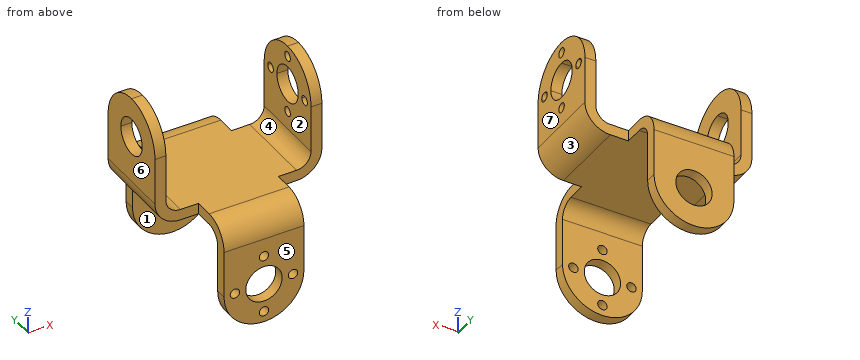
from build123d import *

# Parameters (mm, degrees)
BOSS_EXTRUDE1_DEPTH  = 3
BOSS_EXTRUDE2_DEPTH  = 22
BOSS_EXTRUDE10_DEPTH = 22
BOSS_EXTRUDE3_START  = 3
SKETCH3_R            = 1.3
SKETCH3_R_2          = 5
BOSS_EXTRUDE3_DEPTH  = 3
SKETCH5_W            = 32
SKETCH5_H            = 22
BOSS_EXTRUDE4_DEPTH  = 3
BOSS_EXTRUDE5_DEPTH  = 22
SKETCH8_R            = 1.3
BOSS_EXTRUDE8_DEPTH  = 3
BOSS_EXTRUDE9_START  = -3
BOSS_EXTRUDE9_DEPTH  = 3


with BuildPart() as part:
    # Sketch1 → Boss-Extrude1 (new body)
    with BuildSketch(Plane(origin=(0, 0, 0), x_dir=(1, 0, 0), z_dir=(0, 1, 0))):
        with BuildLine():
            ThreePointArc((-5, 0), (0, 5), (5, 0))
            Line((5, 0), (11, 0))
            ThreePointArc((11, 0), (0, 11), (-11, 0))
            Line((-11, 0), (-5, 0))
        make_face()
        with BuildLine():
            Line((11, 0), (5, 0))
            ThreePointArc((5, 0), (0, -5), (-5, 0))
            Line((-5, 0), (-11, 0))
            ThreePointArc((-11, 0), (0, -11), (11, 0))
        make_face()
        with BuildLine():
            Line((11, -13), (11, 0))
            ThreePointArc((11, 0), (0, -11), (-11, 0))
            Line((-11, 0), (-11, -13))
            Line((-11, -13), (11, -13))
        make_face()
    extrude(amount=BOSS_EXTRUDE1_DEPTH)

    # Sketch2 → Boss-Extrude2 (add)
    with BuildSketch(Plane(origin=(11, 0, 0), x_dir=(0, 0, -1), z_dir=(1, 0, 0))):
        with BuildLine():
            Line((-13, 0), (-13, 3))
            ThreePointArc((-13, 3), (-17.949747468, 0.949747468), (-20, -4))
            Line((-20, -4), (-20, -36))
            Line((-20, -36), (-17, -36))
            Line((-17, -36), (-17, -4))
            ThreePointArc((-17, -4), (-15.828427125, -1.171572875), (-13, 0))
        make_face()
    extrude(amount=-BOSS_EXTRUDE2_DEPTH)

    # Sketch2<4> → Boss-Extrude10 (add)
    with BuildSketch(Plane(origin=(11, 0, 0), x_dir=(0, 0, -1), z_dir=(1, 0, 0))):
        with BuildLine():
            Line((-20, -36), (-17, -36))
            ThreePointArc((-17, -36), (-15.828427125, -38.828427125), (-13, -40))
            Line((-13, -40), (-13, -43))
            ThreePointArc((-13, -43), (-17.949747468, -40.949747468), (-20, -36))
        make_face()
    extrude(amount=-BOSS_EXTRUDE10_DEPTH)

    # Sketch3 → Boss-Extrude3 (add)
    with BuildSketch(Plane(origin=(0, -40, 0), x_dir=(-1, 0, 0), z_dir=(0, -1, 0)).offset(BOSS_EXTRUDE3_START)):
        with BuildLine():
            ThreePointArc((11, 0), (0, 11), (-11, 0))
            Line((-11, 0), (-11, -13))
            Line((-11, -13), (11, -13))
            Line((11, -13), (11, 0))
        make_face()
        with Locations(Location((8, 0, 0), (0, 0, 90))):
            Circle(SKETCH3_R, mode=Mode.SUBTRACT)
        with Locations(Location((0, 0, 0), (0, 0, 270))):
            Circle(SKETCH3_R_2, mode=Mode.SUBTRACT)
        with Locations(Location((-8, 0, 0), (0, 0, 90))):
            Circle(SKETCH3_R, mode=Mode.SUBTRACT)
        with Locations(Location((0, 8, 0), (0, 0, 90))):
            Circle(SKETCH3_R, mode=Mode.SUBTRACT)
        with Locations(Location((0, -8, 0), (0, 0, 90))):
            Circle(SKETCH3_R, mode=Mode.SUBTRACT)
    extrude(amount=-BOSS_EXTRUDE3_DEPTH)

    # Sketch5 → Boss-Extrude4 (add)
    with BuildSketch(Plane.XY.offset(20)):
        with Locations((0, -20)):
            Rectangle(SKETCH5_W, SKETCH5_H)
    extrude(amount=-BOSS_EXTRUDE4_DEPTH)

    # Sketch6 → Boss-Extrude5 (add)
    with BuildSketch(Plane(origin=(0, -9, 0), x_dir=(1, 0, 0), z_dir=(0, 1, 0))):
        with BuildLine():
            Line((-23, -24), (-20, -24))
            ThreePointArc((-20, -24), (-18.828427125, -21.171572875), (-16, -20))
            Line((-16, -20), (-16, -17))
            ThreePointArc((-16, -17), (-20.949747468, -19.050252532), (-23, -24))
        make_face()
        with BuildLine():
            Line((20, -24), (23, -24))
            ThreePointArc((23, -24), (20.949747468, -19.050252532), (16, -17))
            Line((16, -17), (16, -20))
            ThreePointArc((16, -20), (18.828427125, -21.171572875), (20, -24))
        make_face()
    extrude(amount=-BOSS_EXTRUDE5_DEPTH)

    # Sketch8 → Boss-Extrude8 (add)
    # profile 1 of 3: a face of its own
    with BuildSketch(Plane.ZY.offset(-23)):
        with BuildLine():
            Line((37, -9), (24, -9))
            Line((24, -9), (24, -31))
            Line((24, -31), (37, -31))
            ThreePointArc((37, -31), (26, -20), (37, -9))
        make_face()
    # profile 2 of 3: a face of its own
    with BuildSketch(Plane.ZY.offset(-23)):
        with BuildLine():
            Line((37, -10.7), (37, -9))
            ThreePointArc((37, -9), (26, -20), (37, -31))
            Line((37, -31), (37, -29.3))
            ThreePointArc((37, -29.3), (35.7, -28), (37, -26.7))
            Line((37, -26.7), (37, -25))
            ThreePointArc((37, -25), (32, -20), (37, -15))
            Line((37, -15), (37, -13.3))
            ThreePointArc((37, -13.3), (35.7, -12), (37, -10.7))
        make_face()
        with Locations((29, -20)):
            Circle(SKETCH8_R, mode=Mode.SUBTRACT)
    # profile 3 of 3: a face of its own
    with BuildSketch(Plane.ZY.offset(-23)):
        with BuildLine():
            ThreePointArc((48, -20), (44.778174593, -12.221825407), (37, -9))
            Line((37, -9), (37, -10.7))
            ThreePointArc((37, -10.7), (37.919238816, -11.080761184), (38.3, -12))
            ThreePointArc((38.3, -12), (37.919238816, -12.919238816), (37, -13.3))
            Line((37, -13.3), (37, -15))
            ThreePointArc((37, -15), (40.535533906, -16.464466094), (42, -20))
            ThreePointArc((42, -20), (40.535533906, -23.535533906), (37, -25))
            Line((37, -25), (37, -26.7))
            ThreePointArc((37, -26.7), (37.919238816, -27.080761184), (38.3, -28))
            ThreePointArc((38.3, -28), (37.919238816, -28.919238816), (37, -29.3))
            Line((37, -29.3), (37, -31))
            ThreePointArc((37, -31), (44.778174593, -27.778174593), (48, -20))
        make_face()
        with Locations((45, -20)):
            Circle(SKETCH8_R, mode=Mode.SUBTRACT)
    extrude(amount=BOSS_EXTRUDE8_DEPTH)

    # Sketch9 → Boss-Extrude9 (add)
    with BuildSketch(Plane.ZY.offset(23).offset(BOSS_EXTRUDE9_START)):
        with BuildLine():
            Line((24, -9), (24, -31))
            Line((24, -31), (37, -31))
            ThreePointArc((37, -31), (26, -20), (37, -9))
            Line((37, -9), (24, -9))
        make_face()
        with BuildLine():
            ThreePointArc((37, -9), (26, -20), (37, -31))
            Line((37, -31), (37, -25))
            ThreePointArc((37, -25), (32, -20), (37, -15))
            Line((37, -15), (37, -9))
        make_face()
        with BuildLine():
            Line((37, -25), (37, -31))
            ThreePointArc((37, -31), (44.778174593, -27.778174593), (48, -20))
            ThreePointArc((48, -20), (44.778174593, -12.221825407), (37, -9))
            Line((37, -9), (37, -15))
            ThreePointArc((37, -15), (40.535533906, -16.464466094), (42, -20))
            ThreePointArc((42, -20), (40.535533906, -23.535533906), (37, -25))
        make_face()
    extrude(amount=BOSS_EXTRUDE9_DEPTH)


solid = part.part
Build history of the part. All positions in model axes, mm. Face numbers are marked on the shaded views. A direction names the side the tool comes from. Coordinates: 2 decimals unless noted, no trailing zeros. Order: outer loops, then holes, each group sorted by start corner. A loop starts at its lowest first (then second) coordinate and runs counter-clockwise, first axis right, second up. Notation, with made-up numbers: (69, -8) - (103, -8) arc R18 ccw to (103, 16) - close; hole circle Ø2 at (12.25, 82). An arc over 180 degrees is marked (long way). Write item = value, one per line. Start each with the question number.
1) Saw through at D-D on y = -5. Write the cut outline in (x, z).
2) 3-axis set-ups, long thin cutter, end or side, ignore diameter. For the marked faces 1, 2 and 3: which of +Z, -Z, +X, -X, +Y, -Y reach the whole face in a straight line?
3) Two-plate mould, pull along X, no slides. Class the marked faces 4, 5, 6 and 7: pulls with the +X half, pulls with the -X half, needs draft (parallel to the pull), parting line crosses it, or undercut.
4) Saw through at C-C on x = 14.5. Write the cut outline in (y, z), then the cut area to 3 significant figures.
5) Flat gauge pins, fed straight in: pin 1 Ø13 at (x, z) = (-17.5, 22.5) entering from +Y; pin 2 Ø11 at (y, z) = (-18.5, 41.5) entering from -X; pin 3 Ø6.5 at (x, z) = (0.5, 0.5) entering from +Y; pin 4 Ø9.5 at (x, y) = (7.5, -25.5) entering from +Z. Where does each tip first touch, or does it go through?
6) Saw through at A-A on z = 8. Write the cut outline in (x, y), then the cut area to 3 significant figures.
7) Wall check: line 1 along Y through (x, z) = (7.5, -2.5); line 2 along Z through (x, y) = (-2.5, -32); line 3 along X through (y, z) = (-30.5, 37.5). Give the ranges that are in metal, low to high. Write a range as from..to.
8) Saw through at B-B on x = 8. Write the cut outline in (y, z), then the cut area to 3 significant figures.
From the geometry:
q1.outline = (-11, 17) - (11, 17) - (11, 20) - (-11, 20) - close
q2.face_1 = -Z, +X, -X
q2.face_2 = +Z, +Y, -Y
q2.face_3 = -Z, +X, +Y, -Y
q3.face_4 = undercut
q3.face_5 = needs draft
q3.face_6 = pulls with the -X half
q3.face_7 = pulls with the +X half
q4.outline = (-31, 17) - (-9, 17) - (-9, 20) - (-31, 20) - close
q4.area = 66.0 mm^2
q5.pin_1 = -9
q5.pin_2 = -23
q5.pin_3 = through
q5.pin_4 = 20
q6.outline = (-11, -43) - (-1.3, -43) - (-1.3, -40) - (-11, -40) - close; (-11, 0) - (11, 0) - (11, 3) - (-11, 3) - close; (1.3, -43) - (11, -43) - (11, -40) - (1.3, -40) - close
q6.area = 124 mm^2
q7.line_1 = -43..-40, 0..3
q7.line_2 = 17..20
q7.line_3 = -23..-20, 20..23
q8.outline = (-43, -7.55) - (-40, -7.55) - (-40, -1.3) - (-43, -1.3) - close; (-43, 1.3) - (-40, 1.3) - (-40, 13) arc R4 cw to (-36, 17) - (-4, 17) arc R4 cw to (0, 13) - (0, -7.55) - (3, -7.55) - (3, 13) arc R7 ccw to (-4, 20) - (-36, 20) arc R7 ccw to (-43, 13) - close
q8.area = 263 mm^2
